from build123d import *

# Parameters (mm, degrees)
BOSS_EXTRU_1_DEPTH         = 18
ESQUISSE2_R                = 2.3
ENL_V_MAT_EXTRU_1_DEPTH    = 3
ESQUISSE4_R                = 2.3
ENL_V_MAT_EXTRU_2_DEPTH    = 72.05807484
ESQUISSE5_R                = 2.3
ENL_V_MAT_EXTRU_3_DEPTH    = 3
ESQUISSE6_R                = 2.3
ENL_V_MAT_EXTRU_4_DEPTH    = 72.05807484
ESQUISSE7_R                = 4
BOSS_EXTRU_2_DEPTH         = 6
ESQUISSE7_5_R              = 5
ESQUISSE7_5_R_2            = 4
BOSS_EXTRU_3_DEPTH         = 8
R_P_TITION_LIN_AIRE1_COUNT = 8
R_P_TITION_LIN_AIRE1_PITCH = 14
ESQUISSE8_R                = 2
BOSS_EXTRU_4_DEPTH         = 2
R_P_TITION_LIN_AIRE2_COUNT = 8
R_P_TITION_LIN_AIRE2_PITCH = 14
ESQUISSE9_R                = 4.5
BOSS_EXTRU_5_DEPTH         = 20


with BuildPart() as part:
    # Esquisse1 → Boss.-Extru.1 (new body)
    with BuildSketch(Plane.XY):
        with BuildLine():
            Line((-11, -67.5), (11, -67.5))
            ThreePointArc((11, -67.5), (12.414213562, -66.914213562), (13, -65.5))
            Line((13, -65.5), (13, 63.5))
            ThreePointArc((13, 63.5), (11.828427125, 66.328427125), (9, 67.5))
            Line((9, 67.5), (-9, 67.5))
            ThreePointArc((-9, 67.5), (-11.828427125, 66.328427125), (-13, 63.5))
            Line((-13, 63.5), (-13, -65.5))
            ThreePointArc((-13, -65.5), (-12.414213562, -66.914213562), (-11, -67.5))
        make_face()
    extrude(amount=BOSS_EXTRU_1_DEPTH)

    # Esquisse2 → Enl_v. mat.-Extru.1 (cut)
    with BuildSketch(Plane.XY.offset(18)):
        with BuildLine():
            Line((9, 54.8), (19.370645643, 54.8))
            ThreePointArc((19.370645643, 54.8), (22.670645643, 51.5), (19.370645643, 48.2))
            Line((19.370645643, 48.2), (9, 48.2))
            ThreePointArc((9, 48.2), (5.7, 51.5), (9, 54.8))
        make_face()
        with Locations((9, 51.5)):
            Circle(ESQUISSE2_R, mode=Mode.SUBTRACT)
    extrude(amount=-ENL_V_MAT_EXTRU_1_DEPTH, mode=Mode.SUBTRACT)

    # Esquisse4 → Enl_v. mat.-Extru.2 (cut, through all)
    with BuildSketch(Plane.XY.offset(18)):
        with Locations((9, 51.5)):
            Circle(ESQUISSE4_R)
    extrude(amount=-ENL_V_MAT_EXTRU_2_DEPTH, mode=Mode.SUBTRACT)

    # Esquisse5 → Enl_v. mat.-Extru.3 (cut)
    with BuildSketch(Plane.XY.offset(18)):
        with BuildLine():
            Line((-9, -57.8), (-17.299115246, -57.8))
            ThreePointArc((-17.299115246, -57.8), (-20.599115246, -54.5), (-17.299115246, -51.2))
            Line((-17.299115246, -51.2), (-9, -51.2))
            ThreePointArc((-9, -51.2), (-5.7, -54.5), (-9, -57.8))
        make_face()
        with Locations((-9, -54.5)):
            Circle(ESQUISSE5_R, mode=Mode.SUBTRACT)
    extrude(amount=-ENL_V_MAT_EXTRU_3_DEPTH, mode=Mode.SUBTRACT)

    # Esquisse6 → Enl_v. mat.-Extru.4 (cut, through all)
    with BuildSketch(Plane.XY.offset(18)):
        with Locations((-9, -54.5)):
            Circle(ESQUISSE6_R)
    extrude(amount=-ENL_V_MAT_EXTRU_4_DEPTH, mode=Mode.SUBTRACT)

    # Esquisse7 → Boss.-Extru.2 (add)
    with BuildSketch(Plane.XY.offset(18)):
        with Locations(Location((-5, -41.5, 0), (0, 0, 180))):
            Circle(ESQUISSE7_R)
    boss_extru_2 = extrude(amount=BOSS_EXTRU_2_DEPTH)

    # Esquisse7_5 → Boss.-Extru.3 (add)
    with BuildSketch(Plane.XY.offset(18)):
        with Locations(Location((-5, -41.5, 0), (0, 0, 180))):
            Circle(ESQUISSE7_5_R)
        with Locations((-5, -41.5)):
            Circle(ESQUISSE7_5_R_2, mode=Mode.SUBTRACT)
    boss_extru_3 = extrude(amount=BOSS_EXTRU_3_DEPTH)

    # R_p_tition lin_aire1: Boss.-Extru.2, Boss.-Extru.3 ×8
    with Locations(*[(0, i * R_P_TITION_LIN_AIRE1_PITCH, 0) for i in range(1, R_P_TITION_LIN_AIRE1_COUNT)]):
        add(boss_extru_2)
        add(boss_extru_3)

    # Esquisse8 → Boss.-Extru.4 (add)
    with BuildSketch(Plane.XY.offset(18)):
        with Locations(Location((2, -42.5, 0), (0, 0, 180))):
            Circle(ESQUISSE8_R)
    boss_extru_4 = extrude(amount=BOSS_EXTRU_4_DEPTH)

    # R_p_tition lin_aire2: Boss.-Extru.4 ×8
    with Locations(*[(0, i * R_P_TITION_LIN_AIRE2_PITCH, 0) for i in range(1, R_P_TITION_LIN_AIRE2_COUNT)]):
        add(boss_extru_4)

    # Esquisse9 → Boss.-Extru.5 (add)
    with BuildSketch(Plane.XZ.offset(67.5)):
        with Locations(Location((0, 10.336677371, 0), (0, 0, 90))):
            Circle(ESQUISSE9_R)
    extrude(amount=BOSS_EXTRU_5_DEPTH)


solid = part.part
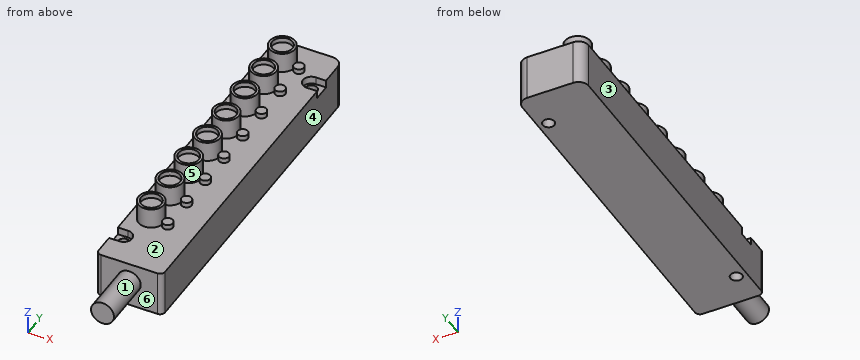
Check sheet for the modelled part. Datum: model origin and axes. Units: mm. Face numbers are marked on the shaded views. A direction names the side the tool comes from. Round coordinates to 2 decimals unless told otherwise and drop trailing zeros. Order: outer loops, then holes, each group sorted by start corner. A loop starts at its lowest first (then second) coordinate and runs counter-clockwise, first axis right, second up.
Q1. Depth check by flat-ended pin: P1, Ø3, axis at x = 3, y = 27.5, coming from the +Z side; P2, Ø8, axis at x = -3, y = -66, coming from the +Z side; P3, Ø1.5, axis at y = -66.5, z = 7.5, coming from the +X side. Enter the tip coordinate at first touch or a pass-through.
Filled sheet:
P1: stops at z = 20
P2: stops at z = 18
P3: stops at x = 12.98
Q2. Draft check along Y on the marked faces 4, 5 and 6. Enter one of: pulls with the +Y half, pulls with the -Y half, needs draft (parallel to the pull), parting line crosses it, or undercut.
Filled sheet:
face 4: needs draft
face 5: undercut
face 6: pulls with the -Y half
Q3. Cross-section at C-C, the plane y = 35.5. Enter the section's corners in (x, z).
Filled sheet:
outline: (-13, 0) - (13, 0) - (13, 18) - (-13, 18) - close
Q4. Cross-section at A-A, the plane y = -54.5. Enter the section's corners in (x, z), plus the area to 3 significant figures.
Filled sheet:
outline: (-13, 0) - (-11.3, 0) - (-11.3, 15) - (-13, 15) - close; (-6.7, 0) - (13, 0) - (13, 18) - (-5.7, 18) - (-5.7, 15) - (-6.7, 15) - close
area: 377 mm2
Q5. Set-up check for the marked faces 1, 2 and 3: record each of +Z, -Z, +X, -X, +Y, -Y from which the full face is reachable in a straight line by a thin tool's end or side.
Filled sheet:
face 1: -Y
face 2: +Z
face 3: +Z, -Z, -X, +Y, -Y
Q6. Cross-section at B-B, the plane z = 9. Enter the section's corners in (x, y).
Filled sheet:
outline: (-13, -65.5) arc R2 ccw to (-11, -67.5) - (-4.3, -67.5) - (-4.3, -87.5) - (4.3, -87.5) - (4.3, -67.5) - (11, -67.5) arc R2 ccw to (13, -65.5) - (13, 63.5) arc R4 ccw to (9, 67.5) - (-9, 67.5) arc R4 ccw to (-13, 63.5) - close; hole circle Ø4.6 at (-9, -54.5); hole circle Ø4.6 at (9, 51.5)
Q7. Scan lines: L1, parallel to Y at x = 9, z = 6.25; L2, parallel to Y at x = -9, z = 10.5; L3, parallel to Z at x = 8.75, y = -15.5. Record each from-to range of solid material in increasing order.
Filled sheet:
L1: y = -67.5 to 49.2, 53.8 to 67.5
L2: y = -67.5 to -56.8, -52.2 to 67.5
L3: z = 0 to 18
